Source: CAD feature listing. Evaluate the final solid. Frame: model axes, mm. A direction names the side the tool comes from. Round coordinates to 2 decimals unless told otherwise and drop trailing zeros. Write each loop counter-clockwise with the first axis right and the second up, starting at its lowest first coordinate (ties: lowest second). Pieces come first, ordered by that corner, then holes.
from build123d import *

# Parameters (mm, degrees)
F0_R     = 8.9154
F1_DEPTH = 25.4
F2_W     = 10.16
F2_H     = 10.16
F3_DEPTH = 10.7696
F4_R     = 3.683
F5_DEPTH = 14.6314
F7_DEPTH = 11.6078
F8_R     = 1.5875
F9_DEPTH = 25.4


with BuildPart() as f1:
    # F0 (on Top) → F1 (new body)
    with BuildSketch(Plane.XY):
        Circle(F0_R)
    extrude(amount=F1_DEPTH)

    # F2 (on face) → F3 (cut)
    with BuildSketch(Plane.XY.offset(25.4)):
        Rectangle(F2_W, F2_H)
    extrude(amount=-F3_DEPTH, mode=Mode.SUBTRACT)

    # F4 (on face) → F5 (cut, through all)
    with BuildSketch(Plane.XY.offset(14.6304)):
        Circle(F4_R)
    extrude(amount=-F5_DEPTH, mode=Mode.SUBTRACT)

    # F6 (on face) → F7 (cut)
    with BuildSketch(Plane(origin=(0, 0, 0), x_dir=(1, 0, 0), z_dir=(0, 0, -1))):
        Polygon((3.739498, 6.477), (-3.739498, 6.477), (-7.478995, 0), (-3.739498, -6.477), (3.739498, -6.477), (7.478995, 0), align=None)
    extrude(amount=-F7_DEPTH, mode=Mode.SUBTRACT)

    # F8 (on face) → F9 (cut, symmetric)
    with BuildSketch(Plane(origin=(0, -6.477, 0), x_dir=(-1, 0, 0), z_dir=(0, 1, 0))):
        with Locations((0.635, 9.7028)):
            Circle(F8_R)
    extrude(amount=F9_DEPTH, both=True, mode=Mode.SUBTRACT)


solid = f1.part
1) Reachability of faces 1 (the face through (0, -5.08, 20)), 2 (the face through (-5.583, -3.284, 5.723)), 3 (the face through (0, -7, 0)) from +Z, -Z, +X, -X, +Y, -Y: full face, straight path, thin tool, end or side. Return the list, or none.
Taken from the geometry:
face 1: +Z
face 2: -Z
face 3: -Z, +X, -X, +Y, -Y
2) Section query C-C on x = 0. Return the cut outline in (y, z).
Taken from the geometry:
outline: (-8.92, 0) - (-6.48, 0) - (-6.48, 8.25) - (-8.92, 8.25) - close; (-8.92, 11.16) - (-6.48, 11.16) - (-6.48, 11.61) - (-3.68, 11.61) - (-3.68, 14.63) - (-5.08, 14.63) - (-5.08, 25.4) - (-8.92, 25.4) - close; (3.68, 11.61) - (6.48, 11.61) - (6.48, 11.16) - (8.92, 11.16) - (8.92, 25.4) - (5.08, 25.4) - (5.08, 14.63) - (3.68, 14.63) - close; (6.48, 0) - (8.92, 0) - (8.92, 8.25) - (6.48, 8.25) - close
3) Contact query for flat-ended pins moving along their axis: P1, Ø3, axis at y = -2, z = 18, coming from the +X side; P2, Ø3, axis at x = 2.5, z = 5, coming from the -Y side; P3, Ø8, axis at x = 6, z = 16, coming from the +Y side. Output: stop coordinate, or through.
Taken from the geometry:
P1: stops at x = 8.9
P2: stops at y = -8.86
P3: stops at y = 8.69
4) Section query D-D on y = 5.5. Return the cut outline in (x, z), then the cut area to 3 significant figures.
Taken from the geometry:
outline: (-7.02, 0) - (-4.3, 0) - (-4.3, 11.61) - (4.3, 11.61) - (4.3, 0) - (7.02, 0) - (7.02, 25.4) - (-7.02, 25.4) - close
area: 257 mm2
5) Section query B-B on y = -0.5. Return the cut outline in (x, z), then the cut area to 3 significant figures.
Taken from the geometry:
outline: (-8.9, 0) - (-7.19, 0) - (-7.19, 11.61) - (-3.65, 11.61) - (-3.65, 14.63) - (-5.08, 14.63) - (-5.08, 25.4) - (-8.9, 25.4) - close; (3.65, 11.61) - (7.19, 11.61) - (7.19, 0) - (8.9, 0) - (8.9, 25.4) - (5.08, 25.4) - (5.08, 14.63) - (3.65, 14.63) - close
area: 154 mm2
6) Material intervals for line 1 (X direction, y = -0.25, z = 17.75); line 2 (Y direction, x = 0, z = 12.4); line 3 (Z direction, x = -2.25, y = -5), sorted ascending.
Taken from the geometry:
line 1: x = -8.91 to -5.08, 5.08 to 8.91
line 2: y = -8.92 to -3.68, 3.68 to 8.92
line 3: z = 11.61 to 14.63
7) Section query A-A on z = 3.5. Return the cut outline in (x, y), then the cut area to 3 significant figures.
Taken from the geometry:
outline: circle Ø17.83 at (0, 0); hole (-7.48, 0) - (-3.74, -6.48) - (3.74, -6.48) - (7.48, 0) - (3.74, 6.48) - (-3.74, 6.48) - close
area: 104 mm2
8) Pull-direction query (X, two-part tool) for faces 4 (the face through (0, -6, 25.4)), 5 (the face through (3, -3, 11.608)), 6 (the face through (2.2, 3.5, 14.63)), 7 (the face through (8.504, 2.678, 12.522)); classes: released by +X, released by -X, zero draft, split by the parting line, or undercut.
Taken from the geometry:
face 4: zero draft
face 5: undercut
face 6: undercut
face 7: split by the parting line
